from build123d import *

# Parameters (mm, degrees)
SKETCH1_R                = 9
SKETCH1_R_2              = 4.25
BOSS_EXTRUDE1_DEPTH      = 40
SKETCH2_R                = 4.9022
CUT_EXTRUDE1_DEPTH       = 10
SKETCH3_R                = 14.693864286
SKETCH3_W                = 14
SKETCH3_H                = 14
CUT_EXTRUDE2_DEPTH       = 40
SKETCH5_R                = 4.5
CUT_EXTRUDE4_DEPTH       = 30
SKETCH14_W               = 8.5
SKETCH14_H               = 8.5
CUT_EXTRUDE10_DEPTH      = 15
FILLET5_R                = 1.5875
CUT_EXTRUDE8_DEPTH       = 25
FILLET6_R                = 0.79375
CIRPATTERN2_COUNT        = 4
FILLET6_OF_CIRPATTERN2_R = 0.79375
FILLET4_R                = 1


with BuildPart() as part:
    # Sketch1 → Boss-Extrude1 (new body)
    with BuildSketch(Plane.XY):
        Circle(SKETCH1_R)
        Circle(SKETCH1_R_2, mode=Mode.SUBTRACT)
    extrude(amount=BOSS_EXTRUDE1_DEPTH)

    # Sketch2 → Cut-Extrude1 (cut)
    with BuildSketch(Plane(origin=(0, 0, 0), x_dir=(-1, 0, 0), z_dir=(0, 0, -1))):
        Circle(SKETCH2_R)
    extrude(amount=-CUT_EXTRUDE1_DEPTH, mode=Mode.SUBTRACT)

    # Sketch3 → Cut-Extrude2 (cut)
    with BuildSketch(Plane(origin=(0, 0, 13), x_dir=(-1, 0, 0), z_dir=(0, 0, -1))):
        Circle(SKETCH3_R)
        Rectangle(SKETCH3_W, SKETCH3_H, mode=Mode.SUBTRACT)
    extrude(amount=-CUT_EXTRUDE2_DEPTH, mode=Mode.SUBTRACT)

    # Sketch5 → Cut-Extrude4 (cut)
    with BuildSketch(Plane(origin=(0, 0, 0), x_dir=(-1, 0, 0), z_dir=(0, 0, -1))):
        Circle(SKETCH5_R)
    extrude(amount=-CUT_EXTRUDE4_DEPTH, mode=Mode.SUBTRACT)

    # Sketch14 → Cut-Extrude10 (cut)
    with BuildSketch(Plane.XY.offset(40)):
        Rectangle(SKETCH14_W, SKETCH14_H)
    extrude(amount=-CUT_EXTRUDE10_DEPTH, mode=Mode.SUBTRACT)

    # Fillet5
    fillet5_edges = [part.edges().sort_by_distance(p)[0] for p in [
        (-4.25, -4.25, 32.5),
        (-4.25, 4.25, 32.5),
        (4.25, 4.25, 32.5),
        (4.25, -4.25, 32.5),
    ]]
    fillet(fillet5_edges, radius=FILLET5_R)

    # Sketch11 → Cut-Extrude8 (cut)
    with BuildSketch(Plane.XY.offset(40)):
        with BuildLine():
            Line((-0.561266008, -0.561266008), (-7.411347572, 6.288815557))
            ThreePointArc((-7.411347572, 6.288815557), (-7.411347572, 7.411347572), (-6.288815557, 7.411347572))
            Line((-6.288815557, 7.411347572), (0.561266008, 0.561266008))
            ThreePointArc((0.561266008, 0.561266008), (0.561266008, -0.561266008), (-0.561266008, -0.561266008))
        make_face()
    cut_extrude8 = extrude(amount=-CUT_EXTRUDE8_DEPTH, mode=Mode.SUBTRACT)

    # Fillet6
    fillet6_edges = [part.edges().sort_by_distance(p)[0] for p in [
        (-4.174359631, 5.296891646, 15),
        (-5.296891646, 4.174359631, 15),
    ]]
    fillet(fillet6_edges, radius=FILLET6_R - 0.0001)  # a hair under: the kernel refuses the full size

    # CirPattern2: Cut-Extrude8 ×4 about axis
    cirpattern2_axis = Axis((0, 0, 0), (0, 0, 1))
    for i in range(1, CIRPATTERN2_COUNT):
        add(cut_extrude8.rotate(cirpattern2_axis, i * 360 / CIRPATTERN2_COUNT), mode=Mode.SUBTRACT)

    # Fillet6 of CirPattern2
    fillet6_of_cirpattern2_edges = [part.edges().sort_by_distance(p)[0] for p in [
        (-5.296891646, -4.174359631, 15),
        (-4.174359631, -5.296891646, 15),
        (4.174359631, -5.296891646, 15),
        (5.296891646, -4.174359631, 15),
        (5.296891646, 4.174359631, 15),
        (4.174359631, 5.296891646, 15),
    ]]
    fillet(fillet6_of_cirpattern2_edges, radius=FILLET6_OF_CIRPATTERN2_R - 0.0001)  # a hair under: the kernel refuses the full size

    # Fillet4
    fillet4_edges = [part.edges().sort_by_distance(p)[0] for p in [
        (-7, 0, 13),
        (0, -7, 13),
        (7, 0, 13),
        (0, 7, 13),
    ]]
    fillet(fillet4_edges, radius=FILLET4_R)


solid = part.part
Check sheet for the modelled part. Datum: model origin and axes. Units: mm. A direction names the side the tool comes from. Coordinates: 2 decimals unless noted, no trailing zeros. Loops run counter-clockwise (first coordinate to the right, second up) from the corner with the lowest first, then second, coordinate; pieces in that order, holes last. Notation, with made-up numbers: (85.25, 37.25) -> (103.25, 37.25) arc R21 ccw to (103.25, 41.25) -> close; hole circle Ø11 at (-0.5, 62.5). An arc over 180 degrees is marked (long way). Write item = value, one per line. Start each with the question number.
1. Section check C-C on z = 23.5. Record the cut outline in (x, y), then the cut area to 3 significant figures.
2. Depth check by flat-ended pin: P1, Ø1, axis at x = -4.5, z = 12.5, coming from the +Y side; P2, Ø6, axis at y = -3.5, z = 11.5, coming from the +X side; P3, Ø8, axis at x = 2.5, z = 29.5, coming from the +Y side. Enter the tip coordinate at first touch or a pass-through.
3. Section check A-A on x = 0. Record the cut outline in (y, z), then the cut area to 3 significant figures.
4. Material ranges on line 1 (X direction, y = 0, z = 22.25); line 2 (X direction, y = -0.5, z = 35.5); line 3 (X direction, y = 5.25, z = 20.5), recorded low to high.
5. Draft check along X on faces 1 (the flat face through (4.2, -5.32, 28.07)), 2 (the flat face through (0, 6, 40)), 3 (the flat face through (-7, 0, 27)). Enter one of: released by +X, released by -X, zero draft, split by the parting line, or undercut.
6. Section check D-D on z = 14.5. Record the cut outline in (x, y).
7. Tool access check on faces 4 (the cylindrical face through (4.378, 5.163, 15.226)), 5 (the cylindrical face through (-4.676, 1.472, 4.93)), 6 (the flat face through (-8.4, 0.1, 13)), 7 (the flat face through (0, 7, 27)). Record the directions out of +Z, -Z, +X, -X, +Y, -Y that give a thin tool (end or side, any length) a straight path to the whole face; none if there is none.
Responses:
q1.outline = (-7, -5.66) arc R9 ccw to (-6.9, -5.78) -> (-3.69, -2.57) arc R4.5 cw to (-3.69, 2.57) -> (-6.9, 5.78) arc R9 ccw to (-7, 5.66) -> close; (-5.78, -6.9) arc R9 ccw to (-5.66, -7) -> (5.66, -7) arc R9 ccw to (5.78, -6.9) -> (2.57, -3.69) arc R4.5 cw to (-2.57, -3.69) -> close; (-5.78, 6.9) -> (-2.57, 3.69) arc R4.5 cw to (2.57, 3.69) -> (5.78, 6.9) arc R9 ccw to (5.66, 7) -> (-5.66, 7) arc R9 ccw to start; (3.69, -2.57) -> (6.9, -5.78) arc R9 ccw to (7, -5.66) -> (7, 5.66) arc R9 ccw to (6.9, 5.78) -> (3.69, 2.57) arc R4.5 cw to start
q1.area = 100 mm2
q2.P1 = 8.06
q2.P2 = 8.99
q2.P3 = 7
q3.outline = (-9, 0) -> (-4.9, 0) -> (-4.9, 10) -> (-4.5, 10) -> (-4.5, 30) -> (-4.25, 30) -> (-4.25, 40) -> (-7, 40) -> (-7, 14) arc R1 cw to (-8, 13) -> (-9, 13) -> close; (4.25, 30) -> (4.5, 30) -> (4.5, 10) -> (4.9, 10) -> (4.9, 0) -> (9, 0) -> (9, 13) -> (8, 13) arc R1 cw to (7, 14) -> (7, 40) -> (4.25, 40) -> close
q3.area = 249 mm2
q4.line_1 = -7 to -4.5, 4.5 to 7
q4.line_2 = -7 to -4.25, 4.25 to 7
q4.line_3 = -7 to -6.37, -4.13 to 4.13, 6.37 to 7
q5.face_1 = undercut
q5.face_2 = zero draft
q5.face_3 = released by -X
q6.outline = (-7, -5.66) arc R9 ccw to (-5.66, -7) -> (5.66, -7) arc R9 ccw to (7, -5.66) -> (7, 5.66) arc R9 ccw to (5.66, 7) -> (-5.66, 7) arc R9 ccw to (-7, 5.66) -> close; hole circle Ø9 at (0, 0)
q7.face_4 = +Z
q7.face_5 = -Z
q7.face_6 = +Z, -X, +Y, -Y
q7.face_7 = +Z, +X, -X, +Y
